from build123d import *

# Parameters (mm, degrees)
EXTRUDE_1_DEPTH = 7.5


with BuildPart() as part:
    # 草图1 → 拉伸-薄壁1 (new body, symmetric)
    with BuildSketch(Plane.XY):
        with BuildLine():
            Line((-16.325, -87.8), (-16.325, 0))
            ThreePointArc((-16.325, 0), (0, 16.325), (16.325, 0))
            Line((16.325, 0), (16.325, -87.8))
            ThreePointArc((16.325, -87.8), (0, -104.125), (-16.325, -87.8))
        make_face()
        with BuildLine():
            Line((-14.325, -87.8), (-14.325, 0))
            ThreePointArc((-14.325, 0), (0, 14.325), (14.325, 0))
            Line((14.325, 0), (14.325, -87.8))
            ThreePointArc((14.325, -87.8), (0, -102.125), (-14.325, -87.8))
        make_face(mode=Mode.SUBTRACT)
    extrude(amount=EXTRUDE_1_DEPTH, both=True)


solid = part.part
The model under review builds one solid part; all positions refer to its coordinate system, in mm. A direction names the side the tool comes from. Give positions to 0.01 mm unless a question says otherwise; leave off trailing zeros. Loops run counter-clockwise (first coordinate to the right, second up) from the corner with the lowest first, then second, coordinate; pieces in that order, holes last. Notation, with made-up numbers: (-23.75, 20) -> (-2.75, 20) arc R22 cw to (-2.75, 55) -> close; hole circle Ø11 at (4, -21.5). An arc over 180 degrees is marked (long way). Answer as a JSON object with one key per item and string values. Group by question number.
Q1. Insertion check: pin 1 (1 mm diameter, centred on x = 2.5, z = -5.5, fed in from +Y); pin 2 (3 mm diameter, centred on y = 4, z = 5, fed in from +X). Each pin has a flat end and moves straight along its axis. Give the tip position at first contact, or say it passes through.
Q2. Take a section at A-A (x = 0). Write out the cut boundary in (y, z) (3 decimals), plus the area to 3 significant figures.
Q3. Wall thickness on line 1 along X through (y, z) = (-52, 4) (3 decimals); line 2 along X through (y, z) = (3, -1.25); line 3 along Y through (x, z) = (-2.5, -2.5): over which ranges is each line inside the solid? List them lowest first.
Q4. Take a section at B-B (y = -5). Write out the cut boundary in (x, z) (3 decimals), plus the area to 3 significant figures.
Q5. Take a section at C-C (z = 3.75). Write out the cut boundary in (x, y) (3 decimals), plus the area to 3 significant figures.
Q6. Draft analysis for pull direction X (two halves, no side actions). For faces 1 (the cylindrical face through (-0.36, 16.32, 0.11)), 2 (the flat face through (14.325, -43, 0)), 3 (the flat face through (-16.325, -45, 0)), state which applies: pulls with the +X half, pulls with the -X half, needs draft (parallel to the pull), parting line crosses it, or undercut.
Q7. Tool access review of faces 4 (the cylindrical face through (0.36, -104.12, 0.11)), 5 (the cylindrical face through (0.31, -102.12, 0.11)): name each direction out of +Z, -Z, +X, -X, +Y, -Y from which nothing blocks a thin tool from reaching the whole face with its end or side.
Answer below:
{
 "1": {"pin 1": "stops at y = 16.2", "pin 2": "stops at x = 16.13"},
 "2": {"outline": "(-104.125, -7.5) -> (-102.125, -7.5) -> (-102.125, 7.5) -> (-104.125, 7.5) -> close; (14.325, -7.5) -> (16.325, -7.5) -> (16.325, 7.5) -> (14.325, 7.5) -> close", "area": "60.0 mm2"},
 "3": {"line 1": "x = -16.325 to -14.325, 14.325 to 16.325", "line 2": "x = -16.05 to -14.01, 14.01 to 16.05", "line 3": "y = -103.93 to -101.91, 14.11 to 16.13"},
 "4": {"outline": "(-16.325, -7.5) -> (-14.325, -7.5) -> (-14.325, 7.5) -> (-16.325, 7.5) -> close; (14.325, -7.5) -> (16.325, -7.5) -> (16.325, 7.5) -> (14.325, 7.5) -> close", "area": "60.0 mm2"},
 "5": {"outline": "(-16.325, -87.8) arc R16.325 ccw to (16.325, -87.8) -> (16.325, 0) arc R16.325 ccw to (-16.325, 0) -> close; hole (-14.325, -87.8) arc R14.325 ccw to (14.325, -87.8) -> (14.325, 0) arc R14.325 ccw to (-14.325, 0) -> close", "area": "544 mm2"},
 "6": {"face 1": "parting line crosses it", "face 2": "undercut", "face 3": "pulls with the -X half"},
 "7": {"face 4": "+Z, -Z, -Y", "face 5": "+Z, -Z"}
}
